from build123d import *

# Parameters (mm, degrees)
F0_W     = 9.5
F0_H     = 10
F1_DEPTH = 20
F2_W     = 3.5
F2_H     = 3
F3_DEPTH = 20
F2_W_2   = 4
F2_H_2   = 2.5
F5_DEPTH = 20
F6_R     = 2
F7_DEPTH = 5
F8_W     = 10
F8_H     = 20
F9_DEPTH = 0.5


# Not quite as in the source:
# - a feature names something its author has since deleted; it is built from what else it names


with BuildPart() as f1:
    # F0 (on Top) → F1 (new body)
    with BuildSketch(Plane.XY):
        with Locations((4.75, 5)):
            Rectangle(F0_W, F0_H)
    extrude(amount=F1_DEPTH)

    # F2 (on face) → F3 (join, through all)
    with BuildSketch(Plane.XY.offset(20)):
        with Locations((-1.75, 5.5)):
            Rectangle(F2_W, F2_H)
    extrude(amount=-F3_DEPTH)

    # F2 (on face) → F5 (join, through all)
    with BuildSketch(Plane.XY.offset(20)):
        with Locations((5, -1.25)):
            Rectangle(F2_W_2, F2_H_2)
    extrude(amount=-F5_DEPTH)

    # F6 (on face) → F7 (join)
    with BuildSketch(Plane(origin=(0, 0, 0), x_dir=(1, 0, 0), z_dir=(0, 0, -1))):
        with Locations((5, -5)):
            Circle(F6_R)
    extrude(amount=F7_DEPTH)

    # F8 (on face) → F9 (join)
    with BuildSketch(Plane.YZ.offset(9.5)):
        with Locations((5, 10)):
            Rectangle(F8_W, F8_H)
    extrude(amount=F9_DEPTH)


solid = f1.part
Source: CAD feature listing. Evaluate the final solid. Frame: model axes, mm. A direction names the side the tool comes from. Give positions to 0.01 mm unless a question says otherwise; leave off trailing zeros. Write each loop counter-clockwise with the first axis right and the second up, starting at its lowest first coordinate (ties: lowest second). Pieces come first, ordered by that corner, then holes. Notation, with made-up numbers: M 66.5,30 L 86.5,30 A28 cw 86.5,59 Z; hole C -18.5,-16 d10. An arc over 180 degrees is marked long. Return JSON: item names as keys, results as strings. Group by question number.
1) Cut plane A-A, the plane z = 15.75. Output: boundary loops of the cut face in (x, y).
2) Material intervals for line 1 along Z through (x, y) = (0.75, 6.5); line 2 along Y through (x, z) = (1.5, 0.75), sorted ascending. Write a range as [from, to].
3) Cut plane C-C, the plane y = 5. Output: boundary loops of the cut face in (x, z), plus the area to 3 significant figures.
4) Pin query (flat end, axial travel): P1, Ø6, axis at x = 8.5, y = 6, coming from the -Z side; P2, Ø3.5, axis at x = 9, z = 5.5, coming from the -Y side; P3, Ø4, axis at x = 7, y = -0.5, coming from the -Z side; P4, Ø0.8, axis at y = -1, z = 7.5, coming from the -X side. Return the tip coordinate at first contact, or that it passes through.
5) Set-up query: faces 1 (the face through (3, -1, 10)), 2 (the face through (8, 0, 10)), 3 (the face through (5, 5, 20)), 4 (the face through (0, 8, 10)), 5 (the face through (3.4, 6.2, -2.5)). Return all of +Z, -Z, +X, -X, +Y, -Y with unobstructed straight access to the full face (end or side cutting, diameter ignored); none if empty.
6) Cut plane B-B, the plane x = 5. Output: boundary loops of the cut face in (y, z), plus the area to 3 significant figures.
7) Cut plane D-D, the plane y = -1. Output: boundary loops of the cut face in (x, z), plus the area to 3 significant figures.
Recorded:
{
 "1": {"outline": "M -3.5,4 L 0,4 L 0,0 L 3,0 L 3,-2.5 L 7,-2.5 L 7,0 L 10,0 L 10,10 L 0,10 L 0,7 L -3.5,7 Z"},
 "2": {"line 1": "z = [0, 20]", "line 2": "y = [0, 10]"},
 "3": {"outline": "M -3.5,0 L 3,0 L 3,-5 L 7,-5 L 7,0 L 10,0 L 10,20 L -3.5,20 Z", "area": "290 mm²"},
 "4": {"P1": "stops at z = -5", "P2": "stops at y = 0", "P3": "stops at z = 0", "P4": "stops at x = 3"},
 "5": {"face 1": "+Z, -Z, -X, -Y", "face 2": "+Z, -Z, +X, -Y", "face 3": "+Z, +X, -X, +Y, -Y", "face 4": "+Z, -Z, -X, +Y", "face 5": "-Z"},
 "6": {"outline": "M -2.5,0 L 3,0 L 3,-5 L 7,-5 L 7,0 L 10,0 L 10,20 L -2.5,20 Z", "area": "270 mm²"},
 "7": {"outline": "M 3,0 L 7,0 L 7,20 L 3,20 Z", "area": "80.0 mm²"}
}
